```python
from build123d import *

# Parameters (mm, degrees)
ESBO_O1_R                = 3.65
RESSALTO_EXTRUS_O1_DEPTH = 1.6
CORTE_EXTRUS_O2_REACH    = 80.982
ESBO_O3_R                = 0.45


with BuildPart() as part:
    # Esboço1 → Ressalto-extrusão1 (new body)
    with BuildSketch(Plane.XY):
        with BuildLine():
            Line((-0.568287769, 9.983839392), (-70.33, 8))
            ThreePointArc((-70.33, 8), (-78.33, 0), (-70.33, -8))
            Line((-70.33, -8), (-0.568287769, -9.983839392))
            Line((-0.568287769, -9.983839392), (0, -10))
            ThreePointArc((0, -10), (10, 0), (0, 10))
            Line((0, 10), (-0.568287769, 9.983839392))
        make_face()
        with Locations((-70.33, 0)):
            Circle(ESBO_O1_R, mode=Mode.SUBTRACT)
        Circle(ESBO_O1_R, mode=Mode.SUBTRACT)
    extrude(amount=RESSALTO_EXTRUS_O1_DEPTH)

    # Esboço3 → Corte-extrusão2 (cut, up to next)
    with BuildSketch(Plane.XY.offset(1.6), mode=Mode.PRIVATE) as corte_extrus_o2_sk1:
        with Locations((-65.65, 0)):
            Circle(ESBO_O3_R)
    corte_extrus_o2_tool1 = extrude(corte_extrus_o2_sk1.sketch, amount=-CORTE_EXTRUS_O2_REACH, mode=Mode.PRIVATE) & part.part
    # Esboço3 → Corte-extrusão2 (cut, up to next)
    with BuildSketch(Plane.XY.offset(1.6), mode=Mode.PRIVATE) as corte_extrus_o2_sk2:
        with Locations((-4.68, 0)):
            Circle(ESBO_O3_R)
    corte_extrus_o2_tool2 = extrude(corte_extrus_o2_sk2.sketch, amount=-CORTE_EXTRUS_O2_REACH, mode=Mode.PRIVATE) & part.part
    # Esboço3 → Corte-extrusão2 (cut, up to next)
    with BuildSketch(Plane.XY.offset(1.6), mode=Mode.PRIVATE) as corte_extrus_o2_sk3:
        with Locations((-6.68, 0)):
            Circle(ESBO_O3_R)
    corte_extrus_o2_tool3 = extrude(corte_extrus_o2_sk3.sketch, amount=-CORTE_EXTRUS_O2_REACH, mode=Mode.PRIVATE) & part.part
    # Esboço3 → Corte-extrusão2 (cut, up to next)
    with BuildSketch(Plane.XY.offset(1.6), mode=Mode.PRIVATE) as corte_extrus_o2_sk4:
        with Locations((-8.68, 0)):
            Circle(ESBO_O3_R)
    corte_extrus_o2_tool4 = extrude(corte_extrus_o2_sk4.sketch, amount=-CORTE_EXTRUS_O2_REACH, mode=Mode.PRIVATE) & part.part
    # Esboço3 → Corte-extrusão2 (cut, up to next)
    with BuildSketch(Plane.XY.offset(1.6), mode=Mode.PRIVATE) as corte_extrus_o2_sk5:
        with Locations((-10.68, 0)):
            Circle(ESBO_O3_R)
    corte_extrus_o2_tool5 = extrude(corte_extrus_o2_sk5.sketch, amount=-CORTE_EXTRUS_O2_REACH, mode=Mode.PRIVATE) & part.part
    # Esboço3 → Corte-extrusão2 (cut, up to next)
    with BuildSketch(Plane.XY.offset(1.6), mode=Mode.PRIVATE) as corte_extrus_o2_sk6:
        with Locations((-12.68, 0)):
            Circle(ESBO_O3_R)
    corte_extrus_o2_tool6 = extrude(corte_extrus_o2_sk6.sketch, amount=-CORTE_EXTRUS_O2_REACH, mode=Mode.PRIVATE) & part.part
    # Esboço3 → Corte-extrusão2 (cut, up to next)
    with BuildSketch(Plane.XY.offset(1.6), mode=Mode.PRIVATE) as corte_extrus_o2_sk7:
        with Locations((-14.68, 0)):
            Circle(ESBO_O3_R)
    corte_extrus_o2_tool7 = extrude(corte_extrus_o2_sk7.sketch, amount=-CORTE_EXTRUS_O2_REACH, mode=Mode.PRIVATE) & part.part
    # Esboço3 → Corte-extrusão2 (cut, up to next)
    with BuildSketch(Plane.XY.offset(1.6), mode=Mode.PRIVATE) as corte_extrus_o2_sk8:
        with Locations((-63.65, 0)):
            Circle(ESBO_O3_R)
    corte_extrus_o2_tool8 = extrude(corte_extrus_o2_sk8.sketch, amount=-CORTE_EXTRUS_O2_REACH, mode=Mode.PRIVATE) & part.part
    # Esboço3 → Corte-extrusão2 (cut, up to next)
    with BuildSketch(Plane.XY.offset(1.6), mode=Mode.PRIVATE) as corte_extrus_o2_sk9:
        with Locations((-61.65, 0)):
            Circle(ESBO_O3_R)
    corte_extrus_o2_tool9 = extrude(corte_extrus_o2_sk9.sketch, amount=-CORTE_EXTRUS_O2_REACH, mode=Mode.PRIVATE) & part.part
    # Esboço3 → Corte-extrusão2 (cut, up to next)
    with BuildSketch(Plane.XY.offset(1.6), mode=Mode.PRIVATE) as corte_extrus_o2_sk10:
        with Locations((-59.65, 0)):
            Circle(ESBO_O3_R)
    corte_extrus_o2_tool10 = extrude(corte_extrus_o2_sk10.sketch, amount=-CORTE_EXTRUS_O2_REACH, mode=Mode.PRIVATE) & part.part
    # Esboço3 → Corte-extrusão2 (cut, up to next)
    with BuildSketch(Plane.XY.offset(1.6), mode=Mode.PRIVATE) as corte_extrus_o2_sk11:
        with Locations((-57.65, 0)):
            Circle(ESBO_O3_R)
    corte_extrus_o2_tool11 = extrude(corte_extrus_o2_sk11.sketch, amount=-CORTE_EXTRUS_O2_REACH, mode=Mode.PRIVATE) & part.part
    # Esboço3 → Corte-extrusão2 (cut, up to next)
    with BuildSketch(Plane.XY.offset(1.6), mode=Mode.PRIVATE) as corte_extrus_o2_sk12:
        with Locations((-55.65, 0)):
            Circle(ESBO_O3_R)
    corte_extrus_o2_tool12 = extrude(corte_extrus_o2_sk12.sketch, amount=-CORTE_EXTRUS_O2_REACH, mode=Mode.PRIVATE) & part.part
    add(corte_extrus_o2_tool1.solids().sort_by_distance((-65.65, 0, 1.6))[0], mode=Mode.SUBTRACT)
    add(corte_extrus_o2_tool2.solids().sort_by_distance((-4.68, 0, 1.6))[0], mode=Mode.SUBTRACT)
    add(corte_extrus_o2_tool3.solids().sort_by_distance((-6.68, 0, 1.6))[0], mode=Mode.SUBTRACT)
    add(corte_extrus_o2_tool4.solids().sort_by_distance((-8.68, 0, 1.6))[0], mode=Mode.SUBTRACT)
    add(corte_extrus_o2_tool5.solids().sort_by_distance((-10.68, 0, 1.6))[0], mode=Mode.SUBTRACT)
    add(corte_extrus_o2_tool6.solids().sort_by_distance((-12.68, 0, 1.6))[0], mode=Mode.SUBTRACT)
    add(corte_extrus_o2_tool7.solids().sort_by_distance((-14.68, 0, 1.6))[0], mode=Mode.SUBTRACT)
    add(corte_extrus_o2_tool8.solids().sort_by_distance((-63.65, 0, 1.6))[0], mode=Mode.SUBTRACT)
    add(corte_extrus_o2_tool9.solids().sort_by_distance((-61.65, 0, 1.6))[0], mode=Mode.SUBTRACT)
    add(corte_extrus_o2_tool10.solids().sort_by_distance((-59.65, 0, 1.6))[0], mode=Mode.SUBTRACT)
    add(corte_extrus_o2_tool11.solids().sort_by_distance((-57.65, 0, 1.6))[0], mode=Mode.SUBTRACT)
    add(corte_extrus_o2_tool12.solids().sort_by_distance((-55.65, 0, 1.6))[0], mode=Mode.SUBTRACT)


solid = part.part
```
For this review, take the finished solid that the model builds, in its own axes (mm). Give positions to 0.01 mm unless a question says otherwise; leave off trailing zeros. Write each loop counter-clockwise with the first axis right and the second up, starting at its lowest first coordinate (ties: lowest second). Pieces come first, ordered by that corner, then holes. Notation, with made-up numbers: M 30,-15.5 L 78,-15.5 A22 cw 78,11.5 Z; hole C 38,52 d5. An arc over 180 degrees is marked long. One line per item, written item: value.
1) Take a section at A-A, the plane z = 0.9. Count the separate pieces of the cut face and the enclosed holes in it, then the cut area to 3 significant figures.
Results are:
separate pieces: 1
enclosed holes: 14
area: 1,430 mm²
2) For line 1 (X direction, y = -1.5, z = 1.4); line 2 (X direction, y = -3, z = 0.2); line 3 (Y direction, x = -73, z = 0.9), list the stretches that pass through material, from the lowest coordinate up. Write a range as from..to.
Results are:
line 1: x = -78.19..-73.66, -67..-3.33, 3.33..9.89
line 2: x = -77.75..-72.41, -68.25..-2.08, 2.08..9.54
line 3: y = -7.54..-2.49, 2.49..7.54
3) Take a section at C-C, the plane x = -26.5. Write out the cut boundary in (y, z).
Results are:
outline: M -9.25,0 L 9.25,0 L 9.25,1.6 L -9.25,1.6 Z
4) The part is to be moulded in two halves that separate along X. For faces 1 (the cylindrical face through (-78.328, 0.176, 0.789)), 2 (the cylindrical face through (3.48, 1.1, 0.79)), 3 (the cylindrical face through (10, 0, 1)), say which applies: +X half, -X half, draft (parallel to the pull), parting line (faces both ways), or undercut.
Results are:
face 1: -X half
face 2: undercut
face 3: +X half
5) Take a section at B-B, the plane y = 6. Write out the cut boundary in (x, z).
Results are:
outline: M -75.62,0 L 8,0 L 8,1.6 L -75.62,1.6 Z
